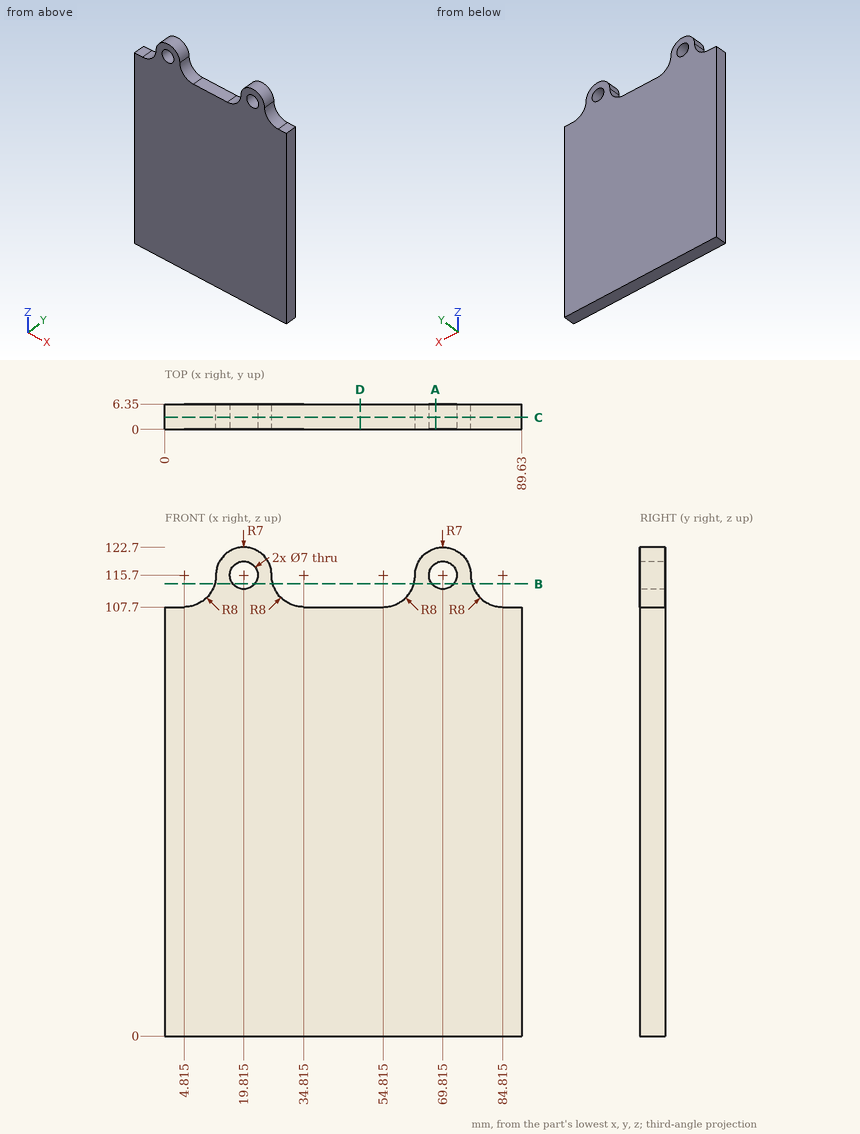
Can you work these out from the drawing? Everything is in mm from the part's minimum corner. Give positions to 0.01 mm unless a question says otherwise; leave off trailing zeros. Loops run counter-clockwise (first coordinate to the right, second up) from the corner with the lowest first, then second, coordinate; pieces in that order, holes last. Notation, with made-up numbers: (2, 12.5) -> (53, 12.5) arc R30 cw to (53, 41.5) -> close; hole circle Ø9 at (56, -2). An arc over 180 degrees is marked (long way). Return JSON: item names as keys, results as strings.
Item 1: If we section it at D-D on x = 49: List the corners of the cut face in (y, z) for me, plus the area to 3 significant figures.
Geometry results:
{"outline": "(0, 0) -> (6.35, 0) -> (6.35, 107.7) -> (0, 107.7) -> close", "area": "684 mm²"}
Item 2: If we section it at C-C on y = 3: List the corners of the cut face in (x, z) for me (3 decimals).
Geometry results:
{"outline": "(0, 0) -> (89.63, 0) -> (89.63, 107.7) -> (84.815, 107.7) arc R8 cw to (76.815, 115.7) arc R7 ccw to (62.815, 115.7) arc R8 cw to (54.815, 107.7) -> (34.815, 107.7) arc R8 cw to (26.815, 115.7) arc R7 ccw to (12.815, 115.7) arc R8 cw to (4.815, 107.7) -> (0, 107.7) -> close; hole circle Ø7 at (19.815, 115.7); hole circle Ø7 at (69.815, 115.7)"}
Item 3: If we section it at B-B on z = 113.5: List the corners of the cut face in (x, y) for me.
Geometry results:
{"outline": "(12.51, 0) -> (17.09, 0) -> (17.09, 6.35) -> (12.51, 6.35) -> close; (22.54, 0) -> (27.12, 0) -> (27.12, 6.35) -> (22.54, 6.35) -> close; (62.51, 0) -> (67.09, 0) -> (67.09, 6.35) -> (62.51, 6.35) -> close; (72.54, 0) -> (77.12, 0) -> (77.12, 6.35) -> (72.54, 6.35) -> close"}
Item 4: If we section it at A-A on x = 68: List the corners of the cut face in (y, z) for me.
Geometry results:
{"outline": "(0, 0) -> (6.35, 0) -> (6.35, 112.71) -> (0, 112.71) -> close; (0, 118.69) -> (6.35, 118.69) -> (6.35, 122.46) -> (0, 122.46) -> close"}
Item 5: I need wall thicknesses on L1, parallel to X at y = 4, z = 115.7 (3 decimals); L2, parallel to X at y = 2, z = 115; L3, parallel to Z at x = 19.5, y = 1.25. Which ranges of each line are inside material? Lowest first, please. Write a range as from..to.
Geometry results:
{"L1": "x = 12.815..16.315, 23.315..26.815, 62.815..66.315, 73.315..76.815", "L2": "x = 12.78..16.39, 23.24..26.85, 62.78..66.39, 73.24..76.85", "L3": "z = 0..112.21, 119.19..122.69"}
